```python
from build123d import *

# Parameters (mm, degrees)
SKETCH_W        = 20
SKETCH_H        = 47.5
PAD_DEPTH       = 12
SKETCH001_R     = 1.6
POCKET_DEPTH    = 8
SKETCH002_R     = 1.6
POCKET001_DEPTH = 8
SKETCH003_W     = 5.8
SKETCH003_H     = 3
POCKET002_DEPTH = 9.5
SKETCH004_R     = 1.6
POCKET003_DEPTH = 12
POCKET004_DEPTH = 9
POCKET005_DEPTH = 50
FILLET_R        = 0.2


with BuildPart() as part:
    # Sketch → Pad (new body)
    with BuildSketch(Plane.XY):
        Rectangle(SKETCH_W, SKETCH_H)
    extrude(amount=PAD_DEPTH)

    # Sketch001 (on Face3 of Pad) → Pocket (cut)
    with BuildSketch(Plane.XZ.offset(23.75)):
        with Locations((-5, 6)):
            Circle(SKETCH001_R)
        with Locations((5, 6)):
            Circle(SKETCH001_R)
    extrude(amount=-POCKET_DEPTH, mode=Mode.SUBTRACT)

    # Sketch002 (on Face1 of Pocket) → Pocket001 (cut)
    with BuildSketch(Plane(origin=(0, 23.75, 0), x_dir=(-1, 0, 0), z_dir=(0, 1, 0))):
        with Locations((-5, 6)):
            Circle(SKETCH002_R)
        with Locations((5, 6)):
            Circle(SKETCH002_R)
    extrude(amount=-POCKET001_DEPTH, mode=Mode.SUBTRACT)

    # Sketch003 (on Face4 of Pocket001) → Pocket002 (cut)
    with BuildSketch(Plane.XY.offset(12)):
        with Locations((-5, 19.25)):
            Rectangle(SKETCH003_W, SKETCH003_H)
        with Locations((5, 19.25)):
            Rectangle(SKETCH003_W, SKETCH003_H)
        with Locations((-5, -19.25)):
            Rectangle(SKETCH003_W, SKETCH003_H)
        with Locations((5, -19.25)):
            Rectangle(SKETCH003_W, SKETCH003_H)
    extrude(amount=-POCKET002_DEPTH, mode=Mode.SUBTRACT)

    # Sketch004 (on Face4 of Pocket002) → Pocket003 (cut)
    with BuildSketch(Plane.XY.offset(12)):
        with Locations((-5, 5)):
            Circle(SKETCH004_R)
        with Locations((5, 5)):
            Circle(SKETCH004_R)
        with Locations((-5, -5)):
            Circle(SKETCH004_R)
        with Locations((5, -5)):
            Circle(SKETCH004_R)
    extrude(amount=-POCKET003_DEPTH, mode=Mode.SUBTRACT)

    # Sketch005 (on Face4 of Pocket003) → Pocket004 (cut)
    with BuildSketch(Plane.XY.offset(12)):
        Polygon((-5, 8.290897), (-7.85, 6.645448), (-7.85, 3.354552), (-5, 1.709103), (-2.15, 3.354552), (-2.15, 6.645448), align=None)
        Polygon((7.85, 6.645448), (5, 8.290897), (2.15, 6.645448), (2.15, 3.354552), (5, 1.709103), (7.85, 3.354552), align=None)
        Polygon((-5, -1.709103), (-7.85, -3.354552), (-7.85, -6.645448), (-5, -8.290897), (-2.15, -6.645448), (-2.15, -3.354552), align=None)
        Polygon((7.85, -3.354552), (5, -1.709103), (2.15, -3.354552), (2.15, -6.645448), (5, -8.290897), (7.85, -6.645448), align=None)
    extrude(amount=-POCKET004_DEPTH, mode=Mode.SUBTRACT)

    # Sketch008 (on Face8 of Pocket004) → Pocket005 (cut)
    with BuildSketch(Plane.XZ.offset(23.75)):
        with BuildLine():
            ThreePointArc((-3, 12), (-7.949747, 9.949747), (-10, 5))
            Line((-10, 5), (-10, 13))
            Line((10, 13), (-10, 13))
            Line((10, 5), (10, 13))
            ThreePointArc((10, 5), (7.949747, 9.949747), (3, 12))
            Line((-3, 12), (3, 12))
        make_face()
    extrude(amount=-POCKET005_DEPTH, mode=Mode.SUBTRACT)

    # Fillet
    fillet_edges = [part.edges().sort_by_distance(p)[0] for p in [
        (10, -23.75, 2.5),
        (-10, -23.75, 2.5),
        (-10, 23.75, 2.5),
        (10, 23.75, 2.5),
    ]]
    fillet(fillet_edges, radius=FILLET_R)


solid = part.part
```
Geometry check sheet. Reference: the model listing, model coordinates, mm. A direction names the side the tool comes from. Give positions to 0.01 mm unless a question says otherwise; leave off trailing zeros. Order: outer loops, then holes, each group sorted by start corner. A loop starts at its lowest first (then second) coordinate and runs counter-clockwise, first axis right, second up. Notation, with made-up numbers: (50, 82) - (72, 82) arc R17 ccw to (72, 114) - close; hole circle Ø6 at (35.25, -6.5). An arc over 180 degrees is marked (long way). Write item = value, one per line. Start each with the question number.
1) Draft check along Y on faces 3 (the flat face through (5, -20.75, 8)), 4 (the flat face through (10, 0, 2)). Enter one of: released by +Y, released by -Y, zero draft, split by the parting line, or undercut.
2) Gauge pin test, flat ends, axial feed: pin 1 Ø6.5 at (x, y) = (4.5, -3.5) entering from +Z; pin 2 Ø1.5 at (y, z) = (19.5, 6.5) entering from +X; pin 3 Ø1.9 at (x, y) = (-5, -5) entering from -Z; pin 4 Ø6 at (x, y) = (-7, 0) entering from +Z. Record the tip position at first contact, or that the pin passes through.
3) Access from +Z, -Z, +X, -X, +Y, -Y to the whole of each face (thin tool, end or side, straight path). Record for faces 1 (the flat face through (0, 0, 12)), 2 (the flat face through (5, 19, 2.5)).
4) Section check A-A (y = -5). Enter the section's corners in (x, z).
5) Scan lines: L1, parallel to Y at x = 5, z = 1.75; L2, parallel to Y at x = -4.25, z = 3.25; L3, parallel to Z at x = -5, y = -22.65. Record each from-to range of solid material in increasing order.
6) Section check B-B (z = 6). Count the separate pieces of the cut face and the enclosed holes in it, then the cut area to 3 significant figures.
Geometry check:
q1.face_3 = undercut
q1.face_4 = zero draft
q2.pin_1 = 12
q2.pin_2 = 9.96
q2.pin_3 = through
q2.pin_4 = 11.93
q3.face_1 = +Z, +X, -X, +Y, -Y
q3.face_2 = +Z
q4.outline = (-10, 0) - (-6.6, 0) - (-6.6, 3) - (-7.85, 3) - (-7.85, 10.05) arc R7 ccw to (-10, 5) - close; (-3.4, 0) - (3.4, 0) - (3.4, 3) - (2.15, 3) - (2.15, 12) - (-2.15, 12) - (-2.15, 3) - (-3.4, 3) - close; (6.6, 0) - (10, 0) - (10, 5) arc R7 ccw to (7.85, 10.05) - (7.85, 3) - (6.6, 3) - close
q5.L1 = -23.75 to -6.6, -3.4 to 3.4, 6.6 to 23.75
q5.L2 = -23.75 to -20.75, -17.75 to -7.86, -2.14 to 2.14, 7.86 to 17.75, 20.75 to 23.75
q5.L3 = 0 to 4.4, 7.6 to 11.71
q6.separate_pieces = 1
q6.enclosed_holes = 4
q6.area = 697 mm2
